Geometry check sheet. Reference: the model listing, model coordinates, mm. A direction names the side the tool comes from. Round coordinates to 2 decimals unless told otherwise and drop trailing zeros. Order: outer loops, then holes, each group sorted by start corner. A loop starts at its lowest first (then second) coordinate and runs counter-clockwise, first axis right, second up.
```python
from build123d import *

# Parameters (mm, degrees)
F2_SIZE   = 0.5
F3_R      = 11
F3_R_2    = 10.5
F4_DEPTH  = 1.5
F6_R      = 11
F6_R_2    = 10.5
F7_DEPTH  = 8.3
F8_SIZE   = 0.5
F11_DEPTH = 25
F12_R     = 3
F13_DEPTH = 12.5


with BuildPart() as f1:
    # F0 (on Front) → F1 (revolve)
    with BuildSketch(Plane.XZ):
        Polygon((0, 4), (0, 0), (32.3, 0), (32.3, 7.5), (23.3, 7.5), (23.3, 10.5), (11.5, 10.5), (11.5, 12), (-12, 12), (-12, 8), (-35.5, 8), (-35.5, 4), align=None)
    revolve(axis=Axis((16.15, 0, 0), (-1, 0, 0)))

    # F2
    f2_edges = [f1.edges().sort_by_distance(p)[0] for p in [
        (-12, 0, -12),
    ]]
    chamfer(f2_edges, length=F2_SIZE)

    # F3 (on face) → F4 (join)
    with BuildSketch(Plane.YZ.offset(23.3)):
        Circle(F3_R)
        Circle(F3_R_2, mode=Mode.SUBTRACT)
    extrude(amount=-F4_DEPTH)

    # F6 (on offset) → F7 (join, through all)
    with BuildSketch(Plane(origin=(19.8, 0, 0), x_dir=(0, -1, 0), z_dir=(-1, 0, 0))):
        Circle(F6_R)
        Circle(F6_R_2, mode=Mode.SUBTRACT)
    extrude(amount=F7_DEPTH)

    # F8
    f8_edges = [f1.edges().sort_by_distance(p)[0] for p in [
        (32.3, 0, -7.5),
        (23.3, -11, 0),
        (11.5, 0, -12),
        (-35.5, 0, -8),
    ]]
    chamfer(f8_edges, length=F8_SIZE)

    # F10 (on offset) → F11 (cut)
    with BuildSketch(Plane.XZ.offset(-7.5)):
        with BuildLine():
            Line((11.5, -3), (16.5, -3))
            ThreePointArc((16.5, -3), (19.5, 0), (16.5, 3))
            Line((16.5, 3), (11.5, 3))
            ThreePointArc((11.5, 3), (8.5, 0), (11.5, -3))
        make_face()
    extrude(amount=-F11_DEPTH, mode=Mode.SUBTRACT)

    # F12 (on Top) → F13 (cut, symmetric)
    with BuildSketch(Plane.XY):
        with Locations((-28, 0)):
            Circle(F12_R)
    extrude(amount=F13_DEPTH, both=True, mode=Mode.SUBTRACT)


solid = f1.part
```
(1) Set-up check for faces 4 (the flat face through (14, 9, 3)), 5 (the flat face through (19.8, -4, -10)), 6 (the flat face through (11.5, -11, -2)): record each of +Z, -Z, +X, -X, +Y, -Y from which the full face is reachable in a straight line by a thin tool's end or side.
Returned:
face 4: +Y
face 5: none
face 6: +X
(2) Sectioned sample at B-B, the plane x = -5. Record the cut outline in (y, z).
Returned:
outline: circle Ø24 at (0, 0); hole circle Ø8 at (0, 0)
(3) Material ranges on line 1 (X direction, y = 0, z = 4.65); line 2 (X direction, y = 10.5, z = 4.25); line 3 (Y direction, x = -28, z = 6.15), recorded low to high.
Returned:
line 1: x = -35.5 to -31, -25 to 32.3
line 2: x = -12 to 11.5
line 3: y = -5.12 to -3, 3 to 5.12
(4) Depth check by flat-ended pin: P1, Ø4, axis at y = 8.5, z = 6, coming from the +X side; P2, Ø9.5, axis at x = -28, y = 0, coming from the +Z side; P3, Ø2.5, axis at x = 13, y = 9.5, coming from the -Z side; P4, Ø12, axis at y = 3.5, z = -9.5, coming from the -X side. Enter the tip coordinate at first touch or a pass-through.
Returned:
P1: stops at x = 23.3
P2: stops at z = 8
P3: stops at z = -7.28
P4: stops at x = -35.5
(5) Sectioned sample at C-C, the plane x = -28. Record the cut outline in (y, z).
Returned:
outline: (-3, -7.42) - (-3, -2.65) arc R4 cw to (-3, 2.65) - (-3, 7.42) arc R8 ccw to start; (3, -7.42) arc R8 ccw to (3, 7.42) - (3, 2.65) arc R4 cw to (3, -2.65) - close
(6) Sectioned sample at A-A, the plane y = 0. Give the number of separate pieces and of enclosed holes in the cut face, and give its area (3 significant figures).
Returned:
separate pieces: 3
enclosed holes: 0
area: 999 mm2
(7) Draft check along X on faces 1 (the flat face through (23.3, 5, -7)), 2 (the flat face through (-35.5, -3, 3)), 3 (the flat face through (14, 7.5, 0)). Enter one of: released by +X, released by -X, zero draft, split by the parting line, or undercut.
Returned:
face 1: released by +X
face 2: released by -X
face 3: undercut
